```python
from build123d import *

# Parameters (mm, degrees)
F0_R          = 127
F0_R_2        = 125.4125
F1_DEPTH      = 254
F2_W          = 279.4
F2_H          = 50.8
F3_DEPTH      = 203.2
F3_DEPTH_BACK = 50.8
F6_DEPTH      = 76.2
F7_R          = 126.9814076924
F8_DEPTH      = 3.175


with BuildPart() as f1:
    # F0 (on Front) → F1 (new body)
    with BuildSketch(Plane.XZ):
        Circle(F0_R)
        Circle(F0_R_2, mode=Mode.SUBTRACT)
    extrude(amount=-F1_DEPTH)

    # F2 (on Top) → F3 (cut, two sides)
    with BuildSketch(Plane.XY) as f3_sk:
        with Locations((0, 76.2)):
            Rectangle(F2_W, F2_H)
    extrude(amount=-F3_DEPTH, mode=Mode.SUBTRACT)
    extrude(f3_sk.sketch, amount=F3_DEPTH_BACK, mode=Mode.SUBTRACT)

    # F5 (on offset) → F6 (cut)
    with BuildSketch(Plane.XY.offset(88.9)):
        Polygon((-50.8, 76.2), (0, 76.2), (50.8, 76.2), (139.7, 203.2), (0, 203.2), (-139.7, 203.2), align=None)
    extrude(amount=F6_DEPTH, mode=Mode.SUBTRACT)

    # F7 (on face) → F8 (join)
    with BuildSketch(Plane(origin=(0, 254, 0), x_dir=(-1, 0, 0), z_dir=(0, 1, 0))):
        Circle(F7_R)
    extrude(amount=F8_DEPTH)


solid = f1.part
```
Read the model definition and answer for the solid it produces. Units are mm, in the model's axes. A direction names the side the tool comes from. Give positions to 0.01 mm unless a question says otherwise; leave off trailing zeros. Write each loop counter-clockwise with the first axis right and the second up, starting at its lowest first coordinate (ties: lowest second). Pieces come first, ordered by that corner, then holes. Notation, with made-up numbers: (-29, 22.5) - (-7, 22.5) arc R17 ccw to (-7, 55.5) - close; hole circle Ø8 at (71, -13.75). An arc over 180 degrees is marked (long way). Write item = value, one per line. Start each with the question number.
Item 1: Find section C-C (y = 29). Give the vertices of the cut face in (x, z) (1 decimal).
Item 2: Find section A-A (x = 0). State how many separate pieces and enclosed holes the cut face has, then the cut area to 3 significant figures.
Item 3: The mould has two halves that part along Z. Classify faces 6 (the cylindrical face through (-100.78, 125.22, -77.28)), 7 (the flat face through (2, 254, 2)), 8 (the flat face through (2, 257.175, 2)): +Z half, -Z half, draft (parallel to the pull), parting line (faces both ways), or undercut.
Item 4: Each of these flat-tipped pins is pushed along its axis until it touches: P1, Ø8, axis at y = 33, z = 50, coming from the +X side; P2, Ø10, axis at x = 41.5, z = -73, coming from the -Y side; P3, Ø0.9, axis at x = 115, y = 66.5, coming from the -Z side. Where does it stop, or does it pass through?
Item 5: A tool of negligible diameter and unlimited length cuts with its end or side. For faces 1 (the cylindrical face through (-99.523, 125.222, -76.312)), 2 (the flat face through (28, 50.8, -123)), 3 (the flat face through (-6, 203.2, 126)), 4 (the cylindrical face through (-121.12, 255.57, 38.14)), 5 (the flat face through (70.65, 104.56, 104.62)), from which of +Z, -Z, +X, -X, +Y, -Y can it reach the whole face along a straight path? Write none if from no direction.
Item 6: Find the intervals of material crossed by probe 1 along X at (y, z) = (116, 0); probe 2 along Y at (x, z) = (-66, -98) (3 decimals); probe 3 along Z at (x, y) = (0, 119), in increasing order. Write a range as [from, to].
Response:
q1.outline = circle Ø254 at (0, 0); hole circle Ø250.8 at (0, 0)
q2.separate_pieces = 3
q2.enclosed_holes = 0
q2.area = 1,330 mm²
q3.face_6 = parting line
q3.face_7 = undercut
q3.face_8 = draft
q4.P1 = 118.38
q4.P2 = 254
q4.P3 = 50.8
q5.face_1 = -Y
q5.face_2 = -Z, +X, -X
q5.face_3 = +Z, +X, -X
q5.face_4 = +Y, -Y
q5.face_5 = +Z
q6.probe_1 = [-127, -125.41], [125.41, 127]
q6.probe_2 = [254, 257.175]
q6.probe_3 = [-127, -125.41]
